Answer from the drawing. Dimensions are ordinates in mm from the lowest x, y and z of the part. Give positions to 0.01 mm unless a question says otherwise; leave off trailing zeros. Write each loop counter-clockwise with the first axis right and the second up, starting at its lowest first coordinate (ties: lowest second). Pieces come first, ordered by that corner, then holes.
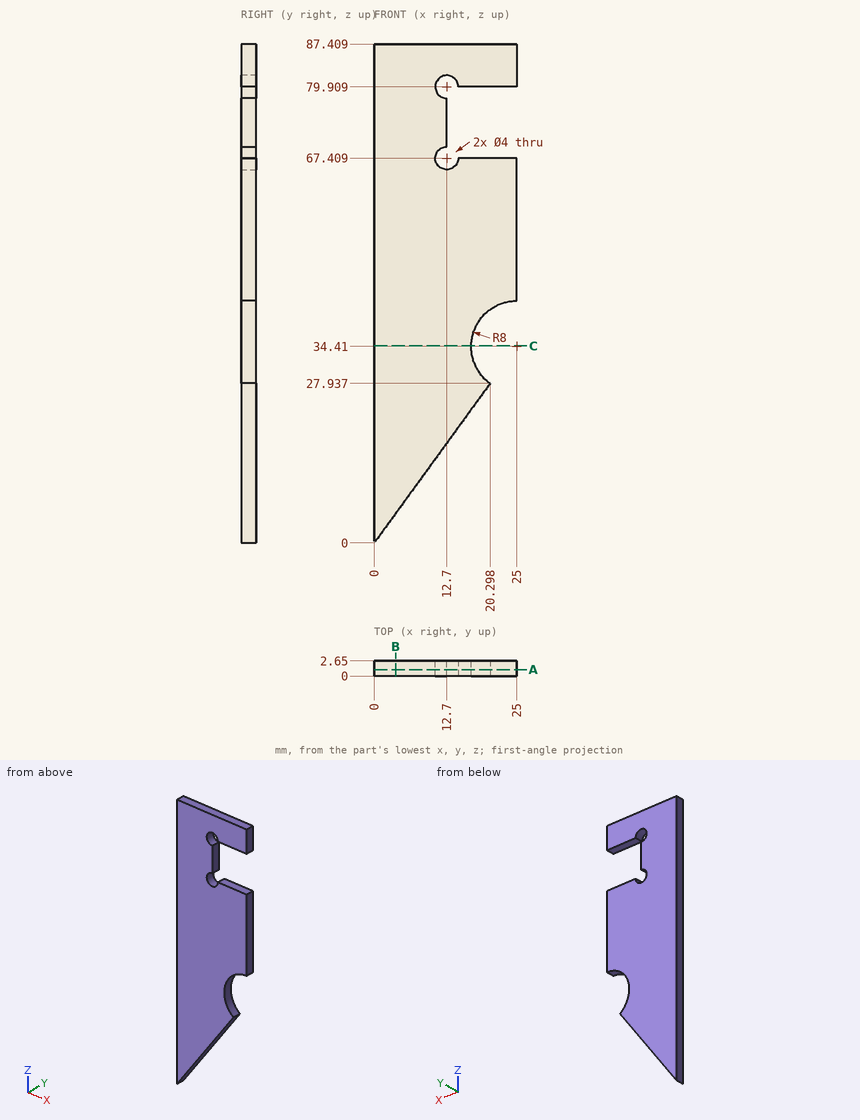
Item 1: Each of these flat-tipped pins is pushed along its axis until it touches: pin 1 Ø1.5 at (x, y) = (6.5, 2) entering from -Z (1 decimal); pin 2 Ø2.5 at (x, z) = (12.7, 79.91) entering from -Y. Where does it stop, or does it pass through?
Result set:
pin 1: stops at z = 7.9
pin 2: passes through
Item 2: Find the intervals of material crossed by line 1 along Z through (x, y) = (14.75, 2.4) (1 decimal); line 2 along Z through (x, y) = (18.5, 0.85) (1 decimal); line 3 along Z through (x, y) = (19.5, 0.6), in increasing order.
Result set:
line 1: z = 20.3 to 67.4, 79.9 to 87.4
line 2: z = 25.5 to 29.7, 39.1 to 67.4, 79.9 to 87.4
line 3: z = 26.84 to 28.6, 40.22 to 67.41, 79.91 to 87.41
Item 3: Section B-B (x = 3.75) is taken. Write down the section's boundary in (y, z), and give its area (3 significant figures).
Result set:
outline: (0, 5.16) - (2.65, 5.16) - (2.65, 87.41) - (0, 87.41) - close
area: 218 mm2
Item 4: Section C-C (z = 34.5) is taken. Write down the section's boundary in (x, y).
Result set:
outline: (0, 0) - (17, 0) - (17, 2.65) - (0, 2.65) - close
Item 5: Section A-A (y = 1.1) is taken. Write down the section's boundary in (x, z), and give its area (3 significant figures).
Result set:
outline: (0, 0) - (20.3, 27.94) arc R8 cw to (25, 42.41) - (25, 67.41) - (14.7, 67.41) arc R2 cw (long way) to (12.7, 69.41) - (12.7, 77.91) arc R2 cw (long way) to (14.7, 79.91) - (25, 79.91) - (25, 87.41) - (0, 87.41) - close
area: 1,500 mm2
